Part model, mm, in its own coordinate system. Face numbers are marked on the shaded views. Give positions to 0.01 mm unless a question says otherwise; leave off trailing zeros. Return JSON: item names as keys, results as strings.
from build123d import *

# Parameters (mm, degrees)
F0_R     = 22.225
F0_R_2   = 20.6375
F1_DEPTH = 25.4
F2_DEPTH = 19.05
F4_D     = 34.925
F5_R     = 1.6002


with BuildPart() as f1:
    # F0 (on Top) → F1 (new body)
    with BuildSketch(Plane.XY):
        Circle(F0_R)
        Circle(F0_R_2, mode=Mode.SUBTRACT)
        Circle(F0_R_2)
    extrude(amount=F1_DEPTH)

    # F0 (on Top) → F2 (cut)
    with BuildSketch(Plane.XY):
        Circle(F0_R_2)
    extrude(amount=F2_DEPTH, mode=Mode.SUBTRACT)

    # F4 (through all)
    with Locations(Plane.XY.offset(25.4)):
        with Locations((0, 0)):
            Hole(F4_D / 2)

    # F5
    f5_edges = [f1.edges().sort_by_distance(p)[0] for p in [
        (-22.225, 0, 25.4),
    ]]
    fillet(f5_edges, radius=F5_R)


solid = f1.part
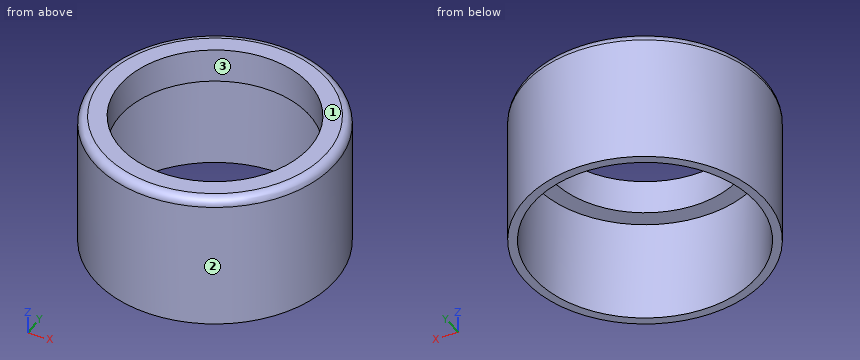
Q1. Two-plate mould, pull along Y, no slides. Class the marked faces 1, 2 and 3: +Y half, -Y half, draft (parallel to the pull), parting line (faces both ways), or undercut.
Established:
{"face 1": "draft", "face 2": "parting line", "face 3": "undercut"}
Q2. Probe line 1 along Y through (x, z) = (0, 22) (1 decimal); line 2 along Y through (x, z) = (0, 8.75) (1 decimal); line 3 along X through (y, z) = (-12, 21.5). List the from-to ranges inside material, lowest first.
Established:
{"line 1": "y = -22.2 to -17.5, 17.5 to 22.2", "line 2": "y = -22.2 to -20.6, 20.6 to 22.2", "line 3": "x = -18.71 to -12.69, 12.69 to 18.71"}
Q3. Pin check, flat tips, straight feed: pin 1 (5 mm diameter, centred on y = 3, z = 15.5, fed in from +X); pin 2 (1.5 mm diameter, centred on x = 16.5, z = 16.5, fed in from -Y); pin 3 (5 mm diameter, centred on y = 11, z = 21, fed in from +X). Stop position of each tip, or through.
Established:
{"pin 1": "stops at x = 22.22", "pin 2": "stops at y = -15.68", "pin 3": "stops at x = 20.54"}
